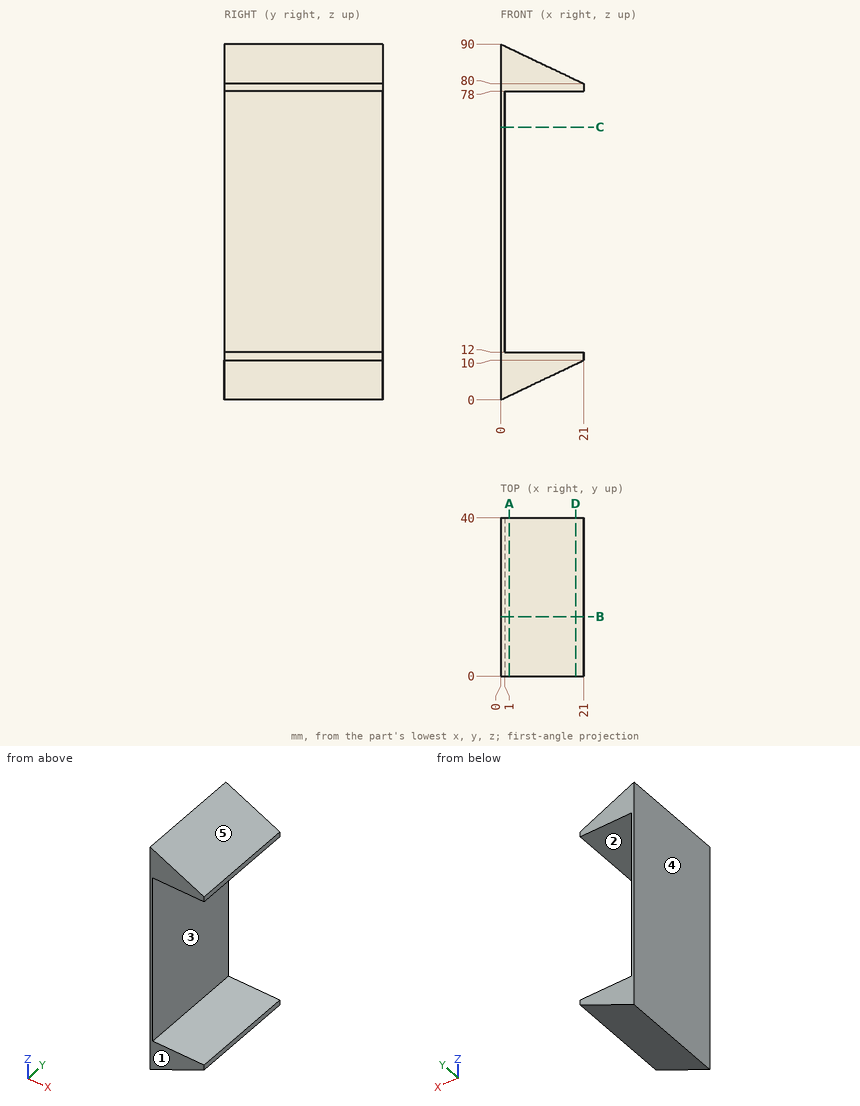
For this review, use the dimensioned drawing (mm, ordinates from the lowest corner) and the shaded views. A direction names the side the tool comes from. Coordinates: 2 decimals unless noted, no trailing zeros. Order: outer loops, then holes, each group sorted by start corner. A loop starts at its lowest first (then second) coordinate and runs counter-clockwise, first axis right, second up. Notation, with made-up numbers: (64, 44.5) -> (83, 44.5) arc R4 ccw to (83, 49.5) -> close; hole circle Ø5 at (67, 25.25). An arc over 180 degrees is marked (long way). One line per item, written item: value. Start each with the question number.
Q1. Take a section at D-D, the plane x = 19. State the section outline as (y, z) points.
Q2. Take a section at B-B, the plane y = 15. State the section outline as (x, z) points, then the cut area to 3 significant figures.
Q3. Take a section at C-C, the plane z = 69. State the section outline as (x, y) points.
Q4. For probe 1 along X at (y, z) = (35.5, 69); probe 2 along Z at (x, y) = (19.25, 19); probe 3 along Z at (x, y) = (9.5, 30), list the stretches that pass through material, from the lowest coordinate up.
Q5. Mouldability with a two-part tool opening along Z and no side actions: class the marked faces 3, 4 and 5 as pulls with the +Z half, pulls with the -Z half, needs draft (parallel to the pull), parting line crosses it, or undercut.
Q6. Insertion check: pin 1 Ø2 at (y, z) = (5, 32.5) entering from +X; pin 2 Ø6 at (x, y) = (9, 5.5) entering from -Z; pin 3 Ø6 at (x, y) = (6, 17.5) entering from +Z. Each pin has a flat end and moves straight along its axis. Give the tip position at first contact, or say it passes through.
Q7. Take a section at A-A, the plane x = 2.25. State the section outline as (y, z) points, then the cut area to 3 significant figures.
Q8. Tool access review of the marked faces 1 and 2: name each direction out of +Z, -Z, +X, -X, +Y, -Y from which nothing blocks a thin tool from reaching the whole face with its end or side.
Values follow:
1. outline: (0, 9.05) -> (40, 9.05) -> (40, 12) -> (0, 12) -> close; (0, 78) -> (40, 78) -> (40, 80.95) -> (0, 80.95) -> close
2. outline: (0, 0) -> (21, 10) -> (21, 12) -> (1, 12) -> (1, 78) -> (21, 78) -> (21, 80) -> (0, 90) -> close
2. area: 360 mm2
3. outline: (0, 0) -> (1, 0) -> (1, 40) -> (0, 40) -> close
4. probe 1: x = 0 to 1
4. probe 2: z = 9.17 to 12, 78 to 80.83
4. probe 3: z = 4.52 to 12, 78 to 85.48
5. face 3: undercut
5. face 4: needs draft
5. face 5: pulls with the +Z half
6. pin 1: stops at x = 1
6. pin 2: stops at z = 2.86
6. pin 3: stops at z = 88.57
7. outline: (0, 1.07) -> (40, 1.07) -> (40, 12) -> (0, 12) -> close; (0, 78) -> (40, 78) -> (40, 88.93) -> (0, 88.93) -> close
7. area: 874 mm2
8. face 1: +Z, -Z, +X, -X, -Y
8. face 2: +X, +Y, -Y
